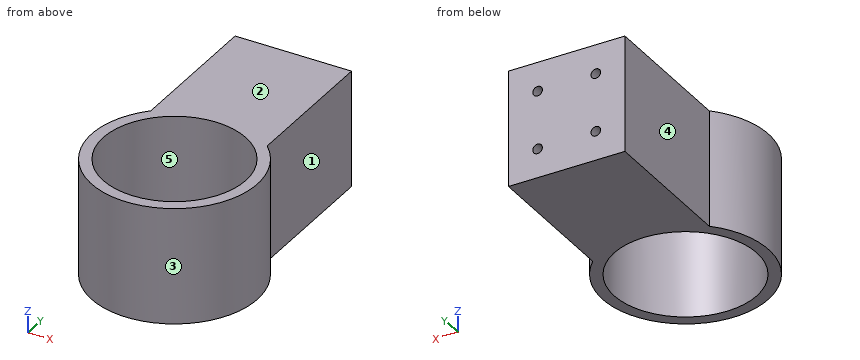
from build123d import *

# Parameters (mm, degrees)
F0_R     = 24.5
F1_DEPTH = 40
F2_R     = 1.65
F3_DEPTH = 35


with BuildPart() as f1:
    # F0 (on Top) → F1 (new body)
    with BuildSketch(Plane.XY):
        with BuildLine():
            Line((20, 70), (-20, 70))
            Line((-20, 70), (-20, 20.303941))
            ThreePointArc((-20, 20.303941), (0, -28.5), (20, 20.303941))
            Line((20, 20.303941), (20, 70))
        make_face()
        Circle(F0_R, mode=Mode.SUBTRACT)
    extrude(amount=F1_DEPTH)

    # F2 (on face) → F3 (cut)
    with BuildSketch(Plane(origin=(0, 70, 0), x_dir=(-1, 0, 0), z_dir=(0, 1, 0))):
        with Locations((-10, 30)):
            Circle(F2_R)
        with Locations((10, 30)):
            Circle(F2_R)
        with Locations((10, 10)):
            Circle(F2_R)
        with Locations((-10, 10)):
            Circle(F2_R)
    extrude(amount=-F3_DEPTH, mode=Mode.SUBTRACT)


solid = f1.part
Here's how the part is built. I have some questions about the finished solid (model axes, mm). Face numbers are marked on the shaded views. A direction names the side the tool comes from. Coordinates: 2 decimals unless noted, no trailing zeros. Write each loop counter-clockwise with the first axis right and the second up, starting at its lowest first coordinate (ties: lowest second). Pieces come first, ordered by that corner, then holes.
1) Thinking about a two-plate mould opening in Y: for the marked faces 3, 4 and 5, which applies, +Y half, -Y half, draft (parallel to the pull), parting line (faces both ways), or undercut?
Filled in:
face 3: parting line
face 4: draft
face 5: undercut
2) If I drill on line 1 (Z direction, x = -10, y = 61); line 2 (Y direction, x = 0, z = 13); line 3 (X direction, y = 49.5, z = 30.5), over which ranges is the centre line in solid material (lowest first)?
Filled in:
line 1: z = 0 to 8.35, 11.65 to 28.35, 31.65 to 40
line 2: y = -28.5 to -24.5, 24.5 to 70
line 3: x = -20 to -11.57, -8.43 to 8.43, 11.57 to 20
3) Which directions (+Z, -Z, +X, -X, +Y, -Y) give clear straight access to the entire face, cutting with the end or side of a thin tool? Please do the marked faces 1 and 2.
Filled in:
face 1: +Z, -Z, +X, +Y
face 2: +Z, +X, -X, +Y, -Y
4) I'm going to push flat-ended pins straight in: pin 1 (2 mm diameter, centred on y = 35.5, z = 5, fed in from -X); pin 2 (2.5 mm diameter, centred on x = 10, z = 10, fed in from +Y); pin 3 (4.5 mm diameter, centred on x = -10, z = 30, fed in from -Y). Where does each tip first touch, or does it pass through?
Filled in:
pin 1: stops at x = -20
pin 2: stops at y = 35
pin 3: stops at y = -27.43
5) If we section it at A-A (y = 63): List the corners of the cut face in (x, z) for me.
Filled in:
outline: (-20, 0) - (20, 0) - (20, 40) - (-20, 40) - close; hole circle Ø3.3 at (-10, 10); hole circle Ø3.3 at (-10, 30); hole circle Ø3.3 at (10, 10); hole circle Ø3.3 at (10, 30)
6) If we section it at C-C (x = 2.5): List the corners of the cut face in (y, z) for me.
Filled in:
outline: (-28.39, 0) - (-24.37, 0) - (-24.37, 40) - (-28.39, 40) - close; (24.37, 0) - (70, 0) - (70, 40) - (24.37, 40) - close
7) If we section it at D-D (y = 9): List the corners of the cut face in (x, z) for me.
Filled in:
outline: (-27.04, 0) - (-22.79, 0) - (-22.79, 40) - (-27.04, 40) - close; (22.79, 0) - (27.04, 0) - (27.04, 40) - (22.79, 40) - close
8) If we section it at B-B (z = 22): List the corners of the cut face in (x, y) for me, plus the area to 3 significant figures.
Filled in:
outline: (-20, 20.3) arc R28.5 ccw (long way) to (20, 20.3) - (20, 70) - (-20, 70) - close; hole circle Ø49 at (0, 0)
area: 2,430 mm2
